Build history of the part. All positions in model axes, mm. Give positions to 0.01 mm unless a question says otherwise; leave off trailing zeros. Order: outer loops, then holes, each group sorted by start corner. A loop starts at its lowest first (then second) coordinate and runs counter-clockwise, first axis right, second up. Notation, with made-up numbers: (-35, 17.5) - (22, 17.5) arc R11 cw to (22, 24.5) - close; hole circle Ø5 at (61, 49). An arc over 180 degrees is marked (long way). Answer in a Markdown table with one row per item.
```python
from build123d import *

# Parameters (mm, degrees)
SKETCH_1_W          = 240
SKETCH_1_H          = 75
EXTRUDE_1_DEPTH     = 1
CHAMFER_1_SIZE      = 10
CUT_EXTRUDE_2_DEPTH = 10
SKETCH_4_R          = 2.1
SKETCH_4_R_2        = 1.6
CUT_EXTRUDE_3_DEPTH = 10
EXTRUDE_2_DEPTH     = 1


with BuildPart() as part:
    # 草图1 → 凸台-拉伸1 (new body)
    with BuildSketch(Plane.XY):
        with Locations((120, 37.5)):
            Rectangle(SKETCH_1_W, SKETCH_1_H)
    extrude(amount=EXTRUDE_1_DEPTH)

    # 倒角1
    chamfer_1_edges = [part.edges().sort_by_distance(p)[0] for p in [
        (0, 75, 0.5),
        (240, 75, 0.5),
        (240, 0, 0.5),
        (0, 0, 0.5),
    ]]
    chamfer(chamfer_1_edges, length=CHAMFER_1_SIZE)

    # 草图3 → 切除-拉伸2 (cut)
    with BuildSketch(Plane(origin=(0, 0, 0), x_dir=(-1, 0, 0), z_dir=(0, 0, -1))):
        Polygon((-148.469655115, 56.990381057), (-135, 33.660254038), (-130, 42.320508076), (-110, 42.320508076), (-105, 33.660254038), (-91.530344885, 56.990381057), (-95, 63), (-145, 63), align=None)
        Polygon((-130, 7.679491924), (-110, 7.679491924), (-100, 25), (-110, 42.320508076), (-130, 42.320508076), (-140, 25), align=None)
    extrude(amount=-CUT_EXTRUDE_2_DEPTH, mode=Mode.SUBTRACT)

    # 草图4 → 切除-拉伸3 (cut)
    with BuildSketch(Plane(origin=(0, 0, 0), x_dir=(-1, 0, 0), z_dir=(0, 0, -1))):
        with Locations((-195, 12)):
            Circle(SKETCH_4_R)
        with Locations((-45, 12)):
            Circle(SKETCH_4_R)
        with Locations((-207.5, 68)):
            Circle(SKETCH_4_R_2)
        with Locations((-192.5, 68)):
            Circle(SKETCH_4_R_2)
        with Locations((-47.5, 68)):
            Circle(SKETCH_4_R_2)
        with Locations((-32.5, 68)):
            Circle(SKETCH_4_R_2)
        with Locations((-235, 37.5)):
            Circle(SKETCH_4_R_2)
        with Locations((-5, 37.5)):
            Circle(SKETCH_4_R_2)
    extrude(amount=-CUT_EXTRUDE_3_DEPTH, mode=Mode.SUBTRACT)

    # 草图5 → 凸台-拉伸2 (add)
    with BuildSketch(Plane.XY.offset(1)):
        Polygon((135, 33.660254038), (123.469655115, 13.689110868), (116.530344885, 13.689110868), (105, 33.660254038), (100, 25), (110, 7.679491924), (130, 7.679491924), (140, 25), align=None)
    extrude(amount=-EXTRUDE_2_DEPTH)


solid = part.part
```
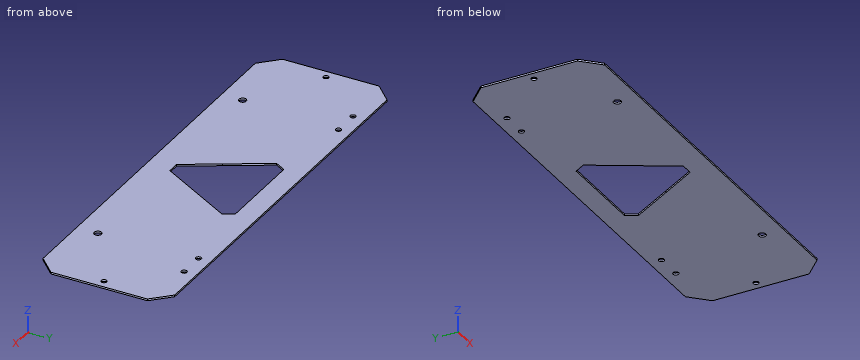
1. Probe line 1 (Y direction, x = 195, z = 0.5); line 2 (X direction, y = 68, z = 0.4); line 3 (Y direction, x = 192.5, z = 0.35). List the from-to ranges inside material, lowest first.
Check result:
| item | result |
|---|---|
| line 1 | y = 0 to 9.9, 14.1 to 75 |
| line 2 | x = 3 to 30.9, 34.1 to 45.9, 49.1 to 190.9, 194.1 to 205.9, 209.1 to 237 |
| line 3 | y = 0 to 66.4, 69.6 to 75 |
2. Drop a flat-ended pin along its axis: P1, Ø2.5, axis at x = 45, y = 12, coming from the -Z side. Give the stop position or say it passes through.
Check result:
| item | result |
|---|---|
| P1 | passes through |
3. Cut at A-A on x = 99. Write the cut outline in (y, z).
Check result:
| item | result |
|---|---|
| outline | (0, 0) - (44.05, 0) - (44.05, 1) - (0, 1) - close; (63, 0) - (75, 0) - (75, 1) - (63, 1) - close |
4. Cut at D-D on y = 7. Write the cut outline in (x, z), and give its area (3 significant figures).
Check result:
| item | result |
|---|---|
| outline | (3, 0) - (237, 0) - (237, 1) - (3, 1) - close |
| area | 234 mm² |
5. Cut at C-C on z = 0.65. Count the separate pieces of the cut face and the enclosed holes in it, and give its area (3 significant figures).
Check result:
| item | result |
|---|---|
| separate pieces | 1 |
| enclosed holes | 9 |
| area | 16,000 mm² |
6. Cut at B-B on y = 60.5. Write the cut outline in (x, z), and give its area (3 significant figures).
Check result:
| item | result |
|---|---|
| outline | (0, 0) - (93.56, 0) - (93.56, 1) - (0, 1) - close; (146.44, 0) - (240, 0) - (240, 1) - (146.44, 1) - close |
| area | 187 mm² |
